```python
from build123d import *

# Parameters (mm, degrees)
BOSS_EXTRUDE1_DEPTH     = 1.5875
SKETCH2_R               = 1.778
CUT_EXTRUDE1_DEPTH      = 1
CUT_EXTRUDE1_DEPTH_BACK = 2.5875


with BuildPart() as part:
    # Sketch1 → Boss-Extrude1 (new body)
    with BuildSketch(Plane(origin=(0, 0, 0), x_dir=(1, 0, 0), z_dir=(0, 1, 0))):
        with BuildLine():
            Line((8.89, -66.675), (43.815, -66.675))
            Line((43.815, -66.675), (43.815, -1.27))
            ThreePointArc((43.815, -1.27), (43.453523156, -0.361476844), (42.545, 0))
            Line((42.545, 0), (-42.545, 0))
            Line((-42.545, 0), (-42.545, -57.785))
            Line((-42.545, -57.785), (-5.08, -57.785))
            ThreePointArc((-5.08, -57.785), (-4.181974388, -58.156974388), (-3.81, -59.055))
            ThreePointArc((-3.81, -59.055), (-3.438025612, -59.953025612), (-2.54, -60.325))
            Line((-2.54, -60.325), (2.54, -60.325))
            Line((2.54, -60.325), (2.54, -73.025))
            ThreePointArc((2.54, -73.025), (4.399871939, -68.534871939), (8.89, -66.675))
        make_face()
    extrude(amount=BOSS_EXTRUDE1_DEPTH)

    # Sketch2 → Cut-Extrude1 (cut, two sides)
    with BuildSketch(Plane(origin=(0, 1.5875, 0), x_dir=(-1, 0, 0), z_dir=(0, 1, 0))) as cut_extrude1_sk:
        with Locations((39.37, 3.175)):
            Circle(SKETCH2_R)
        with Locations((26.035, 3.175)):
            Circle(SKETCH2_R)
        with Locations((12.7, 3.175)):
            Circle(SKETCH2_R)
        with Locations((-0.635, 3.175)):
            Circle(SKETCH2_R)
        with Locations((-13.97, 3.175)):
            Circle(SKETCH2_R)
        with Locations((-27.305, 3.175)):
            Circle(SKETCH2_R)
        with Locations((-40.64, 3.175)):
            Circle(SKETCH2_R)
        with Locations((39.37, 16.03375)):
            Circle(SKETCH2_R)
        with Locations((39.37, 28.8925)):
            Circle(SKETCH2_R)
        with Locations((39.37, 41.75125)):
            Circle(SKETCH2_R)
        with Locations((-40.64, 15.24)):
            Circle(SKETCH2_R)
        with Locations((-40.64, 27.305)):
            Circle(SKETCH2_R)
        with Locations((-40.64, 39.37)):
            Circle(SKETCH2_R)
        with Locations((-40.64, 51.435)):
            Circle(SKETCH2_R)
        with Locations((-40.64, 63.5)):
            Circle(SKETCH2_R)
        with Locations((-24.994404736, 63.5)):
            Circle(SKETCH2_R)
        with Locations((-9.348809473, 63.5)):
            Circle(SKETCH2_R)
        with Locations((-1.889213751, 54.61)):
            Circle(SKETCH2_R)
        with Locations((11.863857499, 54.61)):
            Circle(SKETCH2_R)
        with Locations((25.61692875, 54.61)):
            Circle(SKETCH2_R)
        with Locations((39.37, 54.61)):
            Circle(SKETCH2_R)
    extrude(amount=CUT_EXTRUDE1_DEPTH, mode=Mode.SUBTRACT)
    extrude(cut_extrude1_sk.sketch, amount=-CUT_EXTRUDE1_DEPTH_BACK, mode=Mode.SUBTRACT)


solid = part.part
```
Verification items for the finished model (mm, model axes). Coordinates: 2 decimals unless noted, no trailing zeros. Loops run counter-clockwise (first coordinate to the right, second up) from the corner with the lowest first, then second, coordinate; pieces in that order, holes last. Notation, with made-up numbers: (79.5, 16.25) - (87.5, 16.25) arc R21 ccw to (87.5, 41.25) - close; hole circle Ø10 at (57, 29). An arc over 180 degrees is marked (long way). Answer as a JSON object with one key per item and string values.
(1) Scan lines: line 1 along Z through (x, y) = (-39.37, 0.75) (1 decimal); line 2 along X through (y, z) = (0.8, 28) (3 decimals); line 3 along Z through (x, y) = (30.5, 0.2) (3 decimals). Record each from-to range of solid material in increasing order.
Response:
{"line 1": "z = 0 to 1.4, 5 to 14.3, 17.8 to 27.1, 30.7 to 40, 43.5 to 52.8, 56.4 to 57.8", "line 2": "x = -42.545 to -40.908, -37.832 to 39.003, 42.277 to 43.815", "line 3": "z = 0 to 66.675"}
(2) Mould release check, pull along X, two halves, no side actions. Record for faces 1 (the cylindrical face through (4.351, 0.783, 68.585)), 2 (the cylindrical face through (42.05, 0.8, 26.22)), 3 (the flat face through (0, 0, 28)): pulls with the +X half, pulls with the -X half, needs draft (parallel to the pull), parting line crosses it, or undercut.
Response:
{"face 1": "pulls with the +X half", "face 2": "undercut", "face 3": "needs draft"}
(3) Cross-section at D-D, the plane y = 0.85. Count the separate pieces of the cut face and the enclosed holes in it, then the cut area to 3 significant figures.
Response:
{"separate pieces": "1", "enclosed holes": "21", "area": "5,170 mm²"}
(4) Cross-section at B-B, the plane x = 13.97. Record the boundary of the cut face in (y, z) (1 decimal).
Response:
{"outline": "(0, 0) - (1.6, 0) - (1.6, 1.4) - (0, 1.4) - close; (0, 5) - (1.6, 5) - (1.6, 66.7) - (0, 66.7) - close"}
(5) Cross-section at A-A, the plane z = 54.61. Record the boundary of the cut face in (x, y) (1 decimal), then the cut area to 3 significant figures.
Response:
{"outline": "(-42.5, 0) - (-41.1, 0) - (-41.1, 1.6) - (-42.5, 1.6) - close; (-37.6, 0) - (-27.4, 0) - (-27.4, 1.6) - (-37.6, 1.6) - close; (-23.8, 0) - (-13.6, 0) - (-13.6, 1.6) - (-23.8, 1.6) - close; (-10.1, 0) - (0.1, 0) - (0.1, 1.6) - (-10.1, 1.6) - close; (3.7, 0) - (43.8, 0) - (43.8, 1.6) - (3.7, 1.6) - close", "area": "115 mm²"}
(6) Cross-section at C-C, the plane x = -39.37. Record the boundary of the cut face in (y, z) (1 decimal).
Response:
{"outline": "(0, 0) - (1.6, 0) - (1.6, 1.4) - (0, 1.4) - close; (0, 5) - (1.6, 5) - (1.6, 14.3) - (0, 14.3) - close; (0, 17.8) - (1.6, 17.8) - (1.6, 27.1) - (0, 27.1) - close; (0, 30.7) - (1.6, 30.7) - (1.6, 40) - (0, 40) - close; (0, 43.5) - (1.6, 43.5) - (1.6, 52.8) - (0, 52.8) - close; (0, 56.4) - (1.6, 56.4) - (1.6, 57.8) - (0, 57.8) - close"}
(7) Go/stop test with flat-tipped pins: pin 1 Ø2 at (x, z) = (-25.62, 54.61) entering from +Y; pin 2 Ø0.8 at (x, y) = (-18, 1) entering from +Z (3 decimals). Record where each tip stops, or that it passes through.
Response:
{"pin 1": "passes through", "pin 2": "stops at z = 57.785"}
